```python
from build123d import *

# Parameters (mm, degrees)
SKETCH1_R           = 1.5
BOSS_EXTRUDE1_DEPTH = 2.5
FILLET1_R           = 0.5


with BuildPart() as part:
    # Sketch1 → Boss-Extrude1 (new body)
    with BuildSketch(Plane(origin=(0, 0, 0), x_dir=(1, 0, 0), z_dir=(0, 1, 0))):
        Polygon((-3.175426481, 0), (-1.58771324, -2.75), (1.58771324, -2.75), (3.175426481, 0), (1.58771324, 2.75), (-1.58771324, 2.75), align=None)
        with Locations(Location((0, 0, 0), (0, 0, 270))):
            Circle(SKETCH1_R, mode=Mode.SUBTRACT)
    extrude(amount=BOSS_EXTRUDE1_DEPTH)

    # Fillet1
    fillet1_edges = [part.edges().sort_by_distance(p)[0] for p in [
        (0, 0, -1.5),
        (0, 2.5, -1.5),
    ]]
    fillet(fillet1_edges, radius=FILLET1_R)


solid = part.part
```
The listing builds one solid part. Answer for the finished solid, in the listing's coordinates (mm). Round coordinates to 2 decimals unless told otherwise and drop trailing zeros. Write each loop counter-clockwise with the first axis right and the second up, starting at its lowest first coordinate (ties: lowest second). Pieces come first, ordered by that corner, then holes. Notation, with made-up numbers: (56, 77.25) -> (85, 77.25) arc R10 ccw to (85, 91.25) -> close; hole circle Ø10 at (6, -9). An arc over 180 degrees is marked (long way). Answer as a JSON object with one key per item and string values. Group by question number.
Q1. Determine the mould class of faces 1 (the face through (2.37, 1.232, 1.394)), 2 (the face through (0.45, 1.24, 1.43)), 3 (the face through (-2.39, 1.23, 1.36)) for opening direction X: pulls with the +X half, pulls with the -X half, needs draft (parallel to the pull), parting line crosses it, or undercut.
Q2. Straight lines are drawn through the part: line 1 along X through (y, z) = (2.05, -0.9); line 2 along X through (y, z) = (0.2, -0.75); line 3 along Z through (x, y) = (-1.25, 1.5). For each, find the intervals that lie inside material, in ascending order.
Q3. Section C-C (x = 2.25) is taken. Write down the section's boundary in (y, z).
Q4. Section A-A (y = 0.75) is taken. Write down the section's boundary in (x, z), plus the area to 3 significant figures.
Q5. Section B-B (x = -2.5) is taken. Write down the section's boundary in (y, z).
Q6. This flat-tipped pin is pushed along its axis until it touches: pin 1 Ø2.5 at (x, z) = (0, 0) entering from -Y. Where does it stop, or does it pass through?
Check values:
{
 "1": {"face 1": "pulls with the +X half", "face 2": "undercut", "face 3": "pulls with the -X half"},
 "2": {"line 1": "-2.66 to -1.2, 1.2 to 2.66", "line 2": "-2.74 to -1.41, 1.41 to 2.74", "line 3": "-2.75 to -0.83, 0.83 to 2.75"},
 "3": {"outline": "(0, -1.6) -> (2.5, -1.6) -> (2.5, 1.6) -> (0, 1.6) -> close"},
 "4": {"outline": "(-3.18, 0) -> (-1.59, -2.75) -> (1.59, -2.75) -> (3.18, 0) -> (1.59, 2.75) -> (-1.59, 2.75) -> close; hole circle Ø3 at (0, 0)", "area": "19.1 mm^2"},
 "5": {"outline": "(0, -1.17) -> (2.5, -1.17) -> (2.5, 1.17) -> (0, 1.17) -> close"},
 "6": {"pin 1": "through"}
}
